from build123d import *

# Parameters (mm, degrees)
BOX002_W     = 27
BOX002_H     = 20
BOX002_DEPTH = 10
BOX001_W     = 37
BOX001_H     = 20
BOX001_DEPTH = 10
FILLET001_R  = 1.5
BOX003_W     = 5
BOX003_H     = 20
BOX003_DEPTH = 10
FILLET002_R  = 1.5
BOX_W        = 70
BOX_H        = 20
BOX_DEPTH    = 4
FILLET_R     = 1.5


with BuildPart() as cube002:
    # Box002 → Box002 (new body)
    with BuildSketch(Plane(origin=(35, 0, 4), x_dir=(1, 0, 0), z_dir=(0, 0, 1))):
        with Locations((13.5, 10)):
            Rectangle(BOX002_W, BOX002_H)
    extrude(amount=BOX002_DEPTH)


with BuildPart() as fillet001:
    # Box001 → Box001 (new body)
    with BuildSketch(Plane(origin=(30, 0, 4), x_dir=(1, 0, 0), z_dir=(0, 0, 1))):
        with Locations((18.5, 10)):
            Rectangle(BOX001_W, BOX001_H)
    extrude(amount=BOX001_DEPTH)

    # Cut001: cut Cube002
    add(cube002.part, mode=Mode.SUBTRACT)

    # Fillet001
    fillet001_edges = [fillet001.edges().sort_by_distance(p)[0] for p in [
        (30, 10, 14),
        (35, 10, 14),
        (67, 10, 14),
        (62, 10, 14),
    ]]
    fillet(fillet001_edges, radius=FILLET001_R)


with BuildPart() as fillet002:
    # Box003 → Box003 (new body)
    with BuildSketch(Plane(origin=(25, 0, -10), x_dir=(1, 0, 0), z_dir=(0, 0, 1))):
        with Locations((2.5, 10)):
            Rectangle(BOX003_W, BOX003_H)
    extrude(amount=BOX003_DEPTH)

    # Fillet002
    fillet002_edges = [fillet002.edges().sort_by_distance(p)[0] for p in [
        (25, 10, -10),
        (30, 10, -10),
    ]]
    fillet(fillet002_edges, radius=FILLET002_R)


with BuildPart() as fusion:
    # Box → Box (new body)
    with BuildSketch(Plane.XY):
        with Locations((35, 10)):
            Rectangle(BOX_W, BOX_H)
    extrude(amount=BOX_DEPTH)

    # Fillet
    fillet_edges = [fusion.edges().sort_by_distance(p)[0] for p in [
        (0, 10, 4),
        (0, 10, 0),
        (70, 10, 4),
        (70, 10, 0),
    ]]
    fillet(fillet_edges, radius=FILLET_R)

    # Fusion: union Fillet001, Fillet002
    add(fillet001.part)
    add(fillet002.part)


solid = fusion.part
Can you work these out from the model? Positions are in its coordinate system, mm. A direction names the side the tool comes from. Coordinates: 2 decimals unless noted, no trailing zeros. Write each loop counter-clockwise with the first axis right and the second up, starting at its lowest first coordinate (ties: lowest second). Pieces come first, ordered by that corner, then holes.
Q1. Imagine slicing it at D-D, the plane x = 49. List the corners of the cut face in (y, z) for me, plus the area to 3 significant figures.
Results found:
outline: (0, 0) - (20, 0) - (20, 4) - (0, 4) - close
area: 80.0 mm2
Q2. For P1, Ø1, axis at x = 41.5, y = 7.5, coming from the -Z side; P2, Ø10, axis at y = 9.5, z = -6.5, coming from the +X side; P3, Ø7, axis at y = 13, z = 7, coming from the +X side, each with a flat end and sliding along its axis, tell me the tip position at first contact or that it passes through.
Results found:
P1: stops at z = 0
P2: stops at x = 30
P3: stops at x = 69.62
Q3. Imagine slicing it at B-B, the plane y = 13. List the corners of the cut face in (x, z) for me, plus the area to 3 significant figures.
Results found:
outline: (0, 1.5) arc R1.5 ccw to (1.5, 0) - (25, 0) - (25, -8.5) arc R1.5 ccw to (26.5, -10) - (28.5, -10) arc R1.5 ccw to (30, -8.5) - (30, 0) - (68.5, 0) arc R1.5 ccw to (70, 1.5) - (70, 2.5) arc R1.5 ccw to (68.5, 4) - (67, 4) - (67, 12.5) arc R1.5 ccw to (65.5, 14) - (63.5, 14) arc R1.5 ccw to (62, 12.5) - (62, 4) - (35, 4) - (35, 12.5) arc R1.5 ccw to (33.5, 14) - (31.5, 14) arc R1.5 ccw to (30, 12.5) - (30, 4) - (1.5, 4) arc R1.5 ccw to (0, 2.5) - close
area: 425 mm2
Q4. Imagine slicing it at A-A, the plane z = 8. List the corners of the cut face in (x, y) for me.
Results found:
outline: (30, 0) - (35, 0) - (35, 20) - (30, 20) - close; (62, 0) - (67, 0) - (67, 20) - (62, 20) - close
Q5. If we mould it in two halves opening along X, with no side actions, what happens to faces 1 (the face through (62, 10, 8)), 2 (the face through (0.43, 10.14, 3.55)), 3 (the face through (67, 10, 8))? For each: +X half, -X half, draft (parallel to the pull), parting line (faces both ways), or undercut.
Results found:
face 1: undercut
face 2: -X half
face 3: +X half
Q6. Please list where these lines run through material, in increasing order: L1, parallel to X at y = 6, z = 9; L2, parallel to X at y = 11.5, z = -7.5; L3, parallel to Z at x = 15.5, y = 12.
Results found:
L1: x = 30 to 35, 62 to 67
L2: x = 25 to 30
L3: z = 0 to 4
Q7. Which directions (+Z, -Z, +X, -X, +Y, -Y) give clear straight access to the entire face, cutting with the end or side of a thin tool? Please do faces 4 (the face through (68, 10, 4)), 5 (the face through (16, 10, 4)), 6 (the face through (25, 10, -4)), 7 (the face through (30, 10, -4)), 8 (the face through (48, 10, 4)).
Results found:
face 4: +Z, +X, +Y, -Y
face 5: +Z, -X, +Y, -Y
face 6: -Z, -X, +Y, -Y
face 7: -Z, +X, +Y, -Y
face 8: +Z, +Y, -Y
Q8. Imagine slicing it at C-C, the plane z = -4. List the corners of the cut face in (x, y) for me.
Results found:
outline: (25, 0) - (30, 0) - (30, 20) - (25, 20) - close
